```python
from build123d import *

# Parameters (mm, degrees)
F1_DEPTH = 2.9718


with BuildPart() as f1:
    # F0 (on Front) → F1 (new body)
    with BuildSketch(Plane.XZ):
        Polygon((0, 11.2776), (0, 0), (50.8, 0), (50.8, 11.2776), (45.72, 11.2776), (45.72, 8.1026), (42.545, 8.1026), (42.545, 11.2776), (36.957, 11.2776), (36.957, 14.1224), (42.545, 14.1224), (42.545, 17.2974), (45.72, 17.2974), (45.72, 14.1224), (50.8, 14.1224), (50.8, 25.4), (0, 25.4), (0, 14.1224), (5.08, 14.1224), (5.08, 17.2974), (8.255, 17.2974), (8.255, 14.1224), (13.843, 14.1224), (13.843, 11.2776), (8.255, 11.2776), (8.255, 8.1026), (5.08, 8.1026), (5.08, 11.2776), align=None)
    extrude(amount=-F1_DEPTH)


solid = f1.part
```
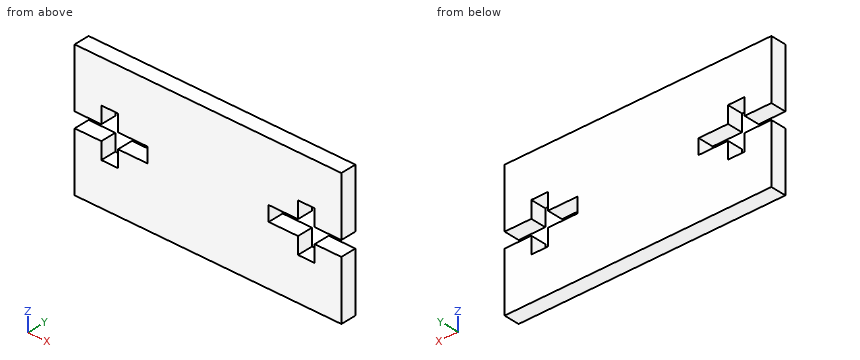
Can you work these out from the model? Positions are in its coordinate system, mm. Coordinates: 2 decimals unless noted, no trailing zeros. Loops run counter-clockwise (first coordinate to the right, second up) from the corner with the lowest first, then second, coordinate; pieces in that order, holes last. Notation, with made-up numbers: (-16.5, 43.5) - (2.5, 43.5) arc R24 cw to (2.5, 59.5) - close; hole circle Ø11 at (-28.75, -12.75). An arc over 180 degrees is marked (long way). Answer as CSV lines item,"result". Start each with the question number.
1) I need wall thicknesses on line 1 (X direction, y = 0.2, z = 9.75) (3 decimals); line 2 (Z direction, x = 2, y = 1.2); line 3 (Z direction, x = 6.5, y = 0.25). Which ranges of each line are inside material? Lowest first, please. Write a range as from..to.
2) Suppose I cut it at D-D (x = 13). Please give me the cut outline in (y, z), plus the area to 3 significant figures.
3) Suppose I cut it at B-B (z = 16.5). Please give me the cut outline in (x, y) (3 decimals), plus the area to 3 significant figures.
4) Suppose I cut it at A-A (x = 7.5). Please give me the cut outline in (y, z).
5) Suppose I cut it at C-C (y = 0.55). Please give me the cut outline in (x, z) (3 decimals), plus the area to 3 significant figures.
Check result:
1,line 1,"x = 0..5.08, 8.255..42.545, 45.72..50.8"
1,line 2,"z = 0..11.28, 14.12..25.4"
1,line 3,"z = 0..8.1, 17.3..25.4"
2,outline,"(0, 0) - (2.97, 0) - (2.97, 11.28) - (0, 11.28) - close; (0, 14.12) - (2.97, 14.12) - (2.97, 25.4) - (0, 25.4) - close"
2,area,"67.0 mm²"
3,outline,"(0, 0) - (5.08, 0) - (5.08, 2.972) - (0, 2.972) - close; (8.255, 0) - (42.545, 0) - (42.545, 2.972) - (8.255, 2.972) - close; (45.72, 0) - (50.8, 0) - (50.8, 2.972) - (45.72, 2.972) - close"
3,area,"132 mm²"
4,outline,"(0, 0) - (2.97, 0) - (2.97, 8.1) - (0, 8.1) - close; (0, 17.3) - (2.97, 17.3) - (2.97, 25.4) - (0, 25.4) - close"
5,outline,"(0, 0) - (50.8, 0) - (50.8, 11.278) - (45.72, 11.278) - (45.72, 8.103) - (42.545, 8.103) - (42.545, 11.278) - (36.957, 11.278) - (36.957, 14.122) - (42.545, 14.122) - (42.545, 17.297) - (45.72, 17.297) - (45.72, 14.122) - (50.8, 14.122) - (50.8, 25.4) - (0, 25.4) - (0, 14.122) - (5.08, 14.122) - (5.08, 17.297) - (8.255, 17.297) - (8.255, 14.122) - (13.843, 14.122) - (13.843, 11.278) - (8.255, 11.278) - (8.255, 8.103) - (5.08, 8.103) - (5.08, 11.278) - (0, 11.278) - close"
5,area,"1,170 mm²"
